Here's how the part is built. I have some questions about the finished solid (model axes, mm). A direction names the side the tool comes from. Give positions to 0.01 mm unless a question says otherwise; leave off trailing zeros. Write each loop counter-clockwise with the first axis right and the second up, starting at its lowest first coordinate (ties: lowest second). Pieces come first, ordered by that corner, then holes. Notation, with made-up numbers: (57.5, -31.75) -> (70.5, -31.75) arc R19 cw to (70.5, -26.75) -> close; hole circle Ø6 at (69, 43). An arc over 180 degrees is marked (long way). Return JSON: item names as keys, results as strings.
from build123d import *

# Parameters (mm, degrees)
EXTRUDE_1_DEPTH     = 47
SKETCH_2_R          = 2.25
CUT_EXTRUDE_1_DEPTH = 90
SKETCH_3_R          = 2.25
CUT_EXTRUDE_2_DEPTH = 40


with BuildPart() as part:
    # 草图1 → 凸台-拉伸1 (new body)
    with BuildSketch(Plane(origin=(0, 0, 0), x_dir=(0, 0, -1), z_dir=(1, 0, 0))):
        with BuildLine():
            Line((0, 0), (350, 0))
            ThreePointArc((350, 0), (375, 25), (350, 50))
            Line((350, 50), (150, 50))
            Line((150, 50), (150, 75))
            Line((150, 75), (350, 75))
            ThreePointArc((350, 75), (400, 25), (350, -25))
            Line((350, -25), (0, -25))
            Line((0, -25), (0, 0))
        make_face()
    extrude(amount=EXTRUDE_1_DEPTH)

    # 草图2 → 切除-拉伸1 (cut)
    with BuildSketch(Plane(origin=(0, 0, 0), x_dir=(1, 0, 0), z_dir=(0, 1, 0))):
        with Locations(Location((36, 15, 0), (0, 0, 270))):
            Circle(SKETCH_2_R)
        with Locations(Location((11, 15, 0), (0, 0, 270))):
            Circle(SKETCH_2_R)
    extrude(amount=-CUT_EXTRUDE_1_DEPTH, mode=Mode.SUBTRACT)

    # 草图3 → 切除-拉伸2 (cut)
    with BuildSketch(Plane(origin=(0, 75, 0), x_dir=(1, 0, 0), z_dir=(0, 1, 0))):
        with Locations(Location((11, 165, 0), (0, 0, 270))):
            Circle(SKETCH_3_R)
        with Locations(Location((36, 165, 0), (0, 0, 270))):
            Circle(SKETCH_3_R)
    extrude(amount=-CUT_EXTRUDE_2_DEPTH, mode=Mode.SUBTRACT)


solid = part.part
1. Suppose I cut it at D-D, the plane y = 25. List the corners of the cut face in (x, z) for me, and give its area (4 significant figures).
Taken from the geometry:
{"outline": "(0, -400) -> (47, -400) -> (47, -375) -> (0, -375) -> close", "area": "1,175 mm²"}
2. If we mould it in two halves opening along Y, with no side actions, what happens to faces 4 (the face through (23, 75, -249)), 5 (the face through (47, -8, -247)), 6 (the face through (23.171, 24.45, -374.994))? For each: released by +Y, released by -Y, zero draft, split by the parting line, or undercut.
Taken from the geometry:
{"face 4": "released by +Y", "face 5": "zero draft", "face 6": "undercut"}
3. If I drill on line 1 (X direction, y = -17, z = -15); line 2 (Y direction, x = 8, z = -345.5); line 3 (Z direction, x = 5, y = 25), over which ranges is the centre line in solid material (lowest first)? Write a range as [from, to].
Taken from the geometry:
{"line 1": "x = [0, 8.75], [13.25, 33.75], [38.25, 47]", "line 2": "y = [-25, 0], [50, 75]", "line 3": "z = [-400, -375]"}
4. For pin 1 Ø3.5 at (x, z) = (11, -15) entering from -Y; pin 2 Ø1 at (x, y) = (12.5, 15) entering from -Z; pin 3 Ø12 at (x, z) = (9, -81) entering from +Y; pin 4 Ø3 at (x, y) = (18, 54) entering from +Z, each with a flat end and sliding along its axis, tell me the tip position at first contact or that it passes through.
Taken from the geometry:
{"pin 1": "passes through", "pin 2": "stops at z = -399.09", "pin 3": "stops at y = 0", "pin 4": "stops at z = -150"}
5. Suppose I cut it at B-B, the plane x = 27. List the corners of the cut face in (y, z) for me.
Taken from the geometry:
{"outline": "(-25, -350) arc R50 ccw to (75, -350) -> (75, -150) -> (50, -150) -> (50, -350) arc R25 cw to (0, -350) -> (0, 0) -> (-25, 0) -> close"}
6. Suppose I cut it at A-A, the plane z = -229.5. List the corners of the cut face in (x, y) for me.
Taken from the geometry:
{"outline": "(0, -25) -> (47, -25) -> (47, 0) -> (0, 0) -> close; (0, 50) -> (47, 50) -> (47, 75) -> (0, 75) -> close"}
7. Suppose I cut it at C-C, the plane z = -64.5. List the corners of the cut face in (x, y) for me.
Taken from the geometry:
{"outline": "(0, -25) -> (47, -25) -> (47, 0) -> (0, 0) -> close"}
8. Which directions (+Z, -Z, +X, -X, +Y, -Y) give clear straight access to the entire face, cutting with the end or side of a thin tool? Please do faces 1 (the face through (23, 62, -150)), 2 (the face through (23, 0, -173)), 3 (the face through (0, -8, -247)).
Taken from the geometry:
{"face 1": "+Z, +X, -X, +Y", "face 2": "+Z, +X, -X", "face 3": "+Z, -Z, -X, +Y, -Y"}
